Read the model definition and answer for the solid it produces. Units are mm, in the model's axes. Face numbers are marked on the shaded views. A direction names the side the tool comes from. Coordinates: 2 decimals unless noted, no trailing zeros. Write each loop counter-clockwise with the first axis right and the second up, starting at its lowest first coordinate (ties: lowest second). Pieces come first, ordered by that corner, then holes.
Item 1: Determine the mould class of the marked faces 1, 2 and 3 for opening direction X: released by +X, released by -X, zero draft, split by the parting line, or undercut.
Item 2: Each of these flat-tipped pins is pushed along its axis until it touches: P1, Ø10, axis at x = 21.5, y = 35.5, coming from the +Z side; P2, Ø2, axis at x = 26.5, z = 50, coming from the -Y side; P3, Ø5, axis at x = 17.5, y = -37, coming from the +Z side; P4, Ø10, axis at x = -11.5, y = -46.5, coming from the -Z side. Where does it stop, or does it pass through?
Item 3: Section A-A (x = 0) is taken. Give the vertices of the cut face in (y, z) (3 decimals).
Item 4: Straight lines are drawn through the part: probe 1 along Y at (x, z) = (0, 8); probe 2 along Z at (x, y) = (44, 2.5); probe 3 along Y at (x, z) = (50, 9). For each, find the intervals that lie inside material, in ascending order.
Item 5: Section B-B (z = 26) is taken. Give the vertices of the cut face in (x, y), then the cut area to 3 significant figures.
Item 6: A tool of negligible diameter and unlimited length cuts with its end or side. For the marked faces 4 and 5, from which of +Z, -Z, +X, -X, +Y, -Y can it reach the whole face along a straight path? Write none if from no direction.
from build123d import *

# Parameters (mm, degrees)
F0_R     = 69.85
F1_DEPTH = 19.05
F2_R     = 35.052
F3_DEPTH = 37.084
F4_R     = 19.05
F5_DEPTH = 56.135
F7_D     = 12.7
F8_R     = 3.175
F9_R     = 5.08


with BuildPart() as f1:
    # F0 (on Top) → F1 (new body)
    with BuildSketch(Plane.XY):
        Circle(F0_R)
    extrude(amount=F1_DEPTH)

    # F2 (on face) → F3 (join)
    with BuildSketch(Plane.XY.offset(19.05)):
        with Locations((0, -1.475124)):
            Circle(F2_R)
    extrude(amount=F3_DEPTH)

    # F4 (on face) → F5 (cut, through all)
    with BuildSketch(Plane.XY.offset(56.134)):
        Circle(F4_R)
    extrude(amount=-F5_DEPTH, mode=Mode.SUBTRACT)

    # F7 (through all)
    with Locations(Plane.XY.offset(19.05)):
        with Locations((0, 53.848), (53.848, 0), (0, -53.848), (-53.848, 0)):
            Hole(F7_D / 2)

    # F8
    f8_edges = [f1.edges().sort_by_distance(p)[0] for p in [
        (-69.85, 0, 19.05),
        (-35.052, -1.475124, 19.05),
    ]]
    fillet(f8_edges, radius=F8_R)

    # F9
    f9_edges = [f1.edges().sort_by_distance(p)[0] for p in [
        (-35.052, -1.475124, 56.134),
    ]]
    fillet(f9_edges, radius=F9_R)


solid = f1.part
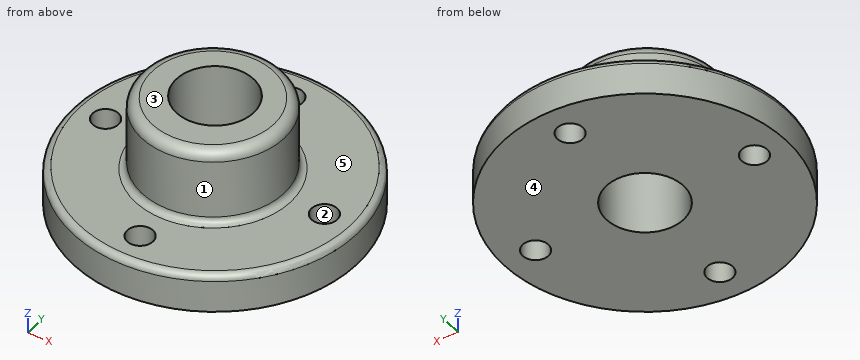
Established:
1. face 1: split by the parting line
1. face 2: undercut
1. face 3: zero draft
2. P1: stops at z = 19.08
2. P2: stops at y = -25.52
2. P3: stops at z = 19.26
2. P4: stops at z = 0
3. outline: (-69.85, 0) - (-60.198, 0) - (-60.198, 19.05) - (-66.675, 19.05) arc R3.175 ccw to (-69.85, 15.875) - close; (-47.498, 0) - (-19.05, 0) - (-19.05, 56.134) - (-31.447, 56.134) arc R5.08 ccw to (-36.527, 51.054) - (-36.527, 22.225) arc R3.175 cw to (-39.702, 19.05) - (-47.498, 19.05) - close; (19.05, 0) - (47.498, 0) - (47.498, 19.05) - (36.752, 19.05) arc R3.175 cw to (33.577, 22.225) - (33.577, 51.054) arc R5.08 ccw to (28.497, 56.134) - (19.05, 56.134) - close; (60.198, 0) - (69.85, 0) - (69.85, 15.875) arc R3.175 ccw to (66.675, 19.05) - (60.198, 19.05) - close
4. probe 1: y = -69.85 to -60.2, -47.5 to -19.05, 19.05 to 47.5, 60.2 to 69.85
4. probe 2: z = 0 to 19.05
4. probe 3: y = -48.78 to -5.05, 5.05 to 48.78
5. outline: circle Ø70.1 at (0, -1.48); hole circle Ø38.1 at (0, 0)
5. area: 2,720 mm2
6. face 4: -Z, +X, -X, +Y, -Y
6. face 5: +Z
